Input: dimensioned drawing with shaded views. Units: mm. Origin: part minimum x, y, z. Coordinates: 2 decimals unless noted, no trailing zeros. Order: outer loops, then holes, each group sorted by start corner. A loop starts at its lowest first (then second) coordinate and runs counter-clockwise, first axis right, second up. Notation, with made-up numbers: (55, 34.25) - (69, 34.25) arc R20 cw to (69, 49.25) - close; hole circle Ø6 at (-32.5, 79). An arc over 180 degrees is marked (long way). Answer as CSV lines item,"result". Start each with the question number.
Item 1: Material intervals for line 1 along Z through (x, y) = (67.5, 0.2); line 2 along Z through (x, y) = (77, 0.55); line 3 along Z through (x, y) = (14, 0.5), sorted ascending.
Item 2: Section B-B (z = 65). Output: boundary loops of the cut face in (x, y).
Item 3: Section D-D (x = 82.5). Output: boundary loops of the cut face in (y, z).
Item 4: Section C-C (z = 92.5). Output: boundary loops of the cut face in (x, y).
Item 5: First-contact query: pin 1 (21 mm diameter, centred on x = 17.37, z = 92.5, fed in from +Y); pin 2 (10 mm diameter, centred on x = 64.5, z = 79.5, fed in from +Y). Flat tips, straight axial feed; report the tip coordinate or a pass-through.
Item 6: Section A-A (x = 65). Output: boundary loops of the cut face in (y, z).
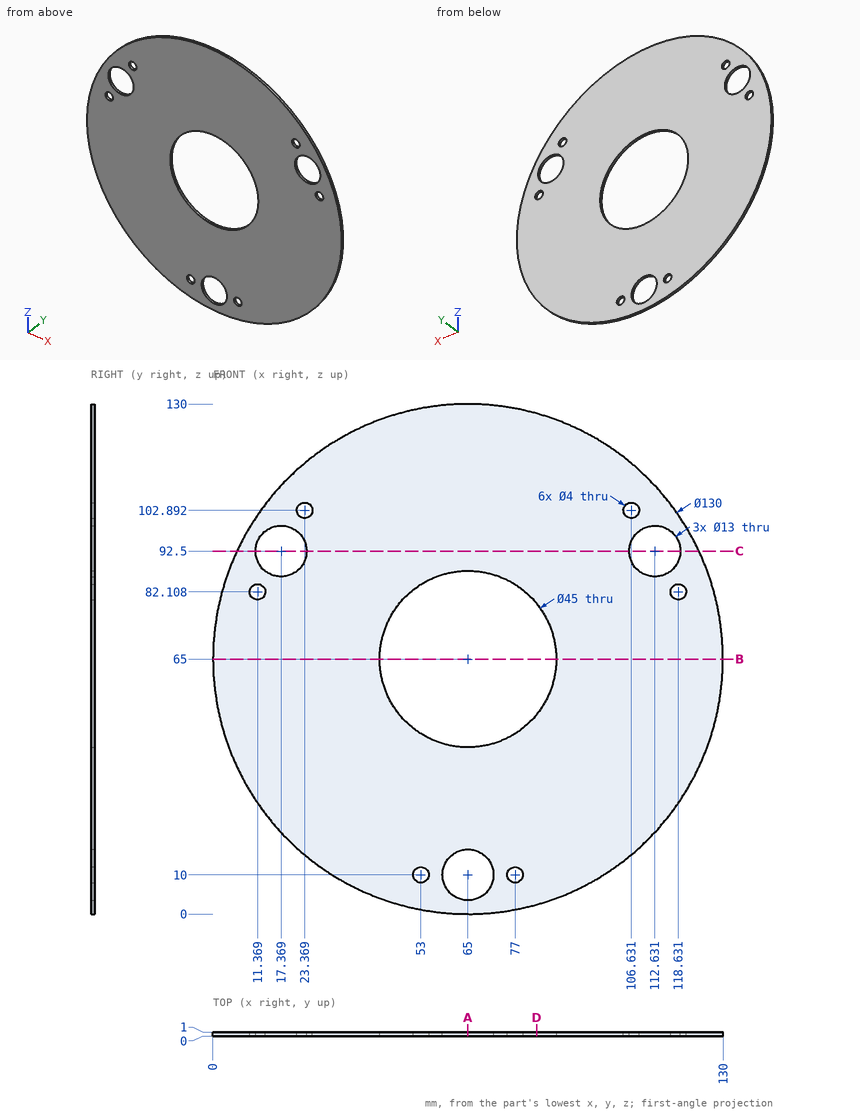
Determined:
1,line 1,"z = 0.05 to 4, 16 to 42.64, 87.36 to 129.95"
1,line 2,"z = 1.12 to 8, 12 to 45.97, 84.03 to 128.88"
1,line 3,"z = 24.7 to 86.94, 98.06 to 105.3"
2,outline,"(0, 0) - (42.5, 0) - (42.5, 1) - (0, 1) - close; (87.5, 0) - (130, 0) - (130, 1) - (87.5, 1) - close"
3,outline,"(0, 2.4) - (1, 2.4) - (1, 50.86) - (0, 50.86) - close; (0, 79.14) - (1, 79.14) - (1, 127.6) - (0, 127.6) - close"
4,outline,"(6.1, 0) - (10.87, 0) - (10.87, 1) - (6.1, 1) - close; (23.87, 0) - (106.13, 0) - (106.13, 1) - (23.87, 1) - close; (119.13, 0) - (123.9, 0) - (123.9, 1) - (119.13, 1) - close"
5,pin 1,"stops at y = 1"
5,pin 2,"passes through"
6,outline,"(0, 0) - (1, 0) - (1, 3.5) - (0, 3.5) - close; (0, 16.5) - (1, 16.5) - (1, 42.5) - (0, 42.5) - close; (0, 87.5) - (1, 87.5) - (1, 130) - (0, 130) - close"
